Design review of the part built by this model. Coordinates are the model's own, in mm. Face numbers are marked on the shaded views. A direction names the side the tool comes from. Coordinates: 2 decimals unless noted, no trailing zeros. Loops run counter-clockwise (first coordinate to the right, second up) from the corner with the lowest first, then second, coordinate; pieces in that order, holes last.
Q1. Machinability: for the marked faces 1, 2 and 3, which of the approach directions +Z, -Z, +X, -X, +Y, -Y give a long, thin tool a straight path to every point of the face, cutting with its end or side? Answer none if there is none.
Q2. Add section C-C on y = 6. Give the boundary of the cut face in (x, z).
Q3. Add section B-B on z = 15. Give the boundary of the cut face in (x, y).
Q4. For P1, Ø0.5, axis at x = 4.5, z = 25.5, coming from the -Y side; P2, Ø5, axis at x = 10.5, z = 24.5, coming from the -Y side; P3, Ø1.5, axis at x = -4, z = 23, coming from the +Y side, all flat-tipped, find the tip position at first contact; note any pin that passes through.
Q5. Add section D-D on x = -5. Give the boundary of the cut face in (y, z), and give its area (3 significant figures).
Q6. Wall thickness on probe 1 along Z at (x, y) = (-1, 9.25); probe 2 along X at (y, z) = (12.5, 25); probe 3 along Z at (x, y) = (2.5, 15.25): over which ranges is each line inside the solid? List them lowest first.
Q7. Add section A-A on y = 14.75. Give the number of separate pieces and of enclosed holes in the cut face, and give its area (3 significant figures).
Q8. Draft analysis for pull direction X (two halves, no side actions). For the marked faces 4, 5 and 6, state which applies: released by +X, released by -X, zero draft, split by the parting line, or undercut.
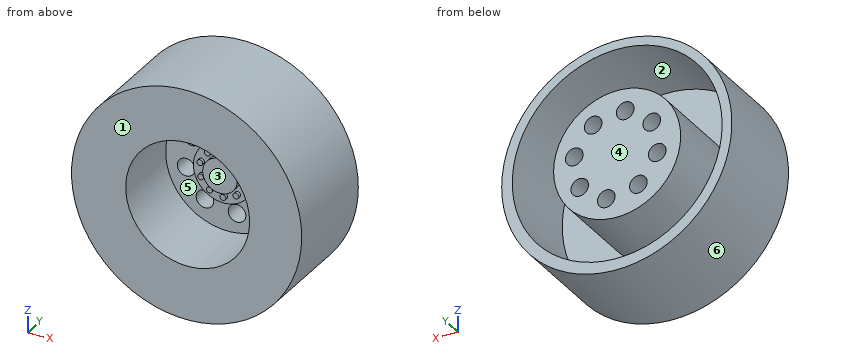
```python
from build123d import *

# Parameters (mm, degrees)
F0_R      = 19.499961
F2_DEPTH  = 16.9999914
F1_R      = 10.5000044
F3_DEPTH  = 12.0000014
F4_R      = 1.4916301958
F5_DEPTH  = 25.4
F7_R      = 17.78
F7_R_2    = 10.7683059636
F8_DEPTH  = 14.9999954
F9_R      = 5.08
F10_DEPTH = 1.27
F13_R     = 2.9336630642
F14_DEPTH = 1.016
F15_R     = 0.4966201378
F16_DEPTH = 0.508


# Not quite as in the source:
# - the program builds the solid bodies; features that only make, move or delete a surface that nothing else refers to are left out


with BuildPart() as f2:
    # F0 (on Front) → F2 (new body)
    with BuildSketch(Plane.XZ):
        with Locations((8.1280004233, 26.7970003188)):
            Circle(F0_R)
    extrude(amount=-F2_DEPTH)

    # F1 (on face) → F3 (cut)
    with BuildSketch(Plane.XZ):
        with Locations((8.3016715726, 26.9168310782)):
            Circle(F1_R)
    extrude(amount=-F3_DEPTH, mode=Mode.SUBTRACT)

    # F4 (on face) → F5 (cut)
    with BuildSketch(Plane.XZ.offset(-12.0000014)):
        with Locations((6.6975592636, 33.9452400804)):
            Circle(F4_R)
        with Locations((12.1372285474, 33.0209454361)):
            Circle(F4_R)
        with Locations((15.3300805747, 28.5209433873)):
            Circle(F4_R)
        with Locations((14.4057859305, 23.0812741034)):
            Circle(F4_R)
        with Locations((9.9057838817, 19.8884220761)):
            Circle(F4_R)
        with Locations((4.4661145978, 20.8127167204)):
            Circle(F4_R)
        with Locations((1.2732625705, 25.3127187692)):
            Circle(F4_R)
        with Locations((2.1975572148, 30.7523880531)):
            Circle(F4_R)
    extrude(amount=-F5_DEPTH, mode=Mode.SUBTRACT)

    # F7 (on face) → F8 (cut)
    with BuildSketch(Plane(origin=(0, 16.9999914, 0), x_dir=(-1, 0, 0), z_dir=(0, 1, 0))):
        with Locations((-8.0529511662, 27.0102884156)):
            Circle(F7_R)
        with Locations((-8.0660926178, 26.997640729)):
            Circle(F7_R_2, mode=Mode.SUBTRACT)
    extrude(amount=-F8_DEPTH, mode=Mode.SUBTRACT)

    # F9 (on face) → F10 (join)
    with BuildSketch(Plane.XZ.offset(-12.0000014)):
        with Locations((8.3016715726, 26.9168310782)):
            Circle(F9_R)
    extrude(amount=F10_DEPTH)

    # F13 (on face) → F14 (join)
    with BuildSketch(Plane.XZ.offset(-10.7300014)):
        with Locations((8.3016715726, 26.9168310782)):
            Circle(F13_R)
    extrude(amount=F14_DEPTH)

    # F15 (on face) → F16 (join)
    with BuildSketch(Plane.XZ.offset(-10.7300014)):
        with Locations((8.092216216, 30.7409893721)):
            Circle(F15_R)
        with Locations((10.3800024772, 30.1337548968)):
            Circle(F15_R)
        with Locations((11.8739369726, 28.297764862)):
            Circle(F15_R)
        with Locations((12.0033875021, 25.934305058)):
            Circle(F15_R)
        with Locations((10.7189083633, 23.9461367989)):
            Circle(F15_R)
        with Locations((8.5111269292, 23.0926727844)):
            Circle(F15_R)
        with Locations((6.2233406681, 23.6999072597)):
            Circle(F15_R)
        with Locations((4.7294061726, 25.5358972945)):
            Circle(F15_R)
        with Locations((4.5999556431, 27.8993570985)):
            Circle(F15_R)
        with Locations((5.884434782, 29.8875253576)):
            Circle(F15_R)
    extrude(amount=F16_DEPTH)


solid = f2.part
```
Entries:
1. face 1: +Z, -Z, +X, -X, -Y
1. face 2: +Y
1. face 3: -Y
2. outline: circle Ø39 at (8.13, 26.8); circle Ø21.54 at (8.07, 27); hole circle Ø35.56 at (8.05, 27.01); hole circle Ø21 at (8.3, 26.92)
3. outline: (-7.4, 0) - (23.65, 0) - (23.65, 17) - (21.16, 17) - (21.16, 2) - (-5.06, 2) - (-5.06, 17) - (-7.4, 17) - close
4. P1: stops at y = 10.22
4. P2: stops at y = 9.71
4. P3: stops at y = 2
5. outline: (0, 12.38) - (17, 12.38) - (17, 14.94) - (2, 14.94) - (2, 39.08) - (17, 39.08) - (17, 41.22) - (0, 41.22) - close
5. area: 128 mm2
6. probe 1: z = 9.57 to 11.71, 21.19 to 22.05, 31.79 to 32.81, 42.31 to 44.03
6. probe 2: x = -11.29 to -9.61, -2.52 to -0.19, 2.73 to 18.65, 25.72 to 27.54
6. probe 3: z = 8.13 to 10.12, 17.78 to 24.46, 26.16 to 29.29, 32.21 to 36.22, 43.9 to 45.47
7. separate pieces: 2
7. enclosed holes: 9
7. area: 510 mm2
8. face 4: zero draft
8. face 5: undercut
8. face 6: split by the parting line
